```python
from build123d import *

# Parameters (mm, degrees)
SKETCH020_W             = 25.4
SKETCH020_H             = 3.175
PAD005_DEPTH            = 25.4
SKETCH001_W             = 28.575
SKETCH001_H             = 10.16
PAD006_DEPTH            = 1.81
PAD006_DEPTH_BACK       = 4.445
POCKET004_DEPTH         = 9.525
POCKET005_DEPTH         = 12.7
CHAMFER_SIZE            = 1.8034
SKETCH023_R             = 3.2512
POCKET006_DEPTH         = 4.446
PAD007_DEPTH            = 10.795
FILLET_R                = 5.08
BODY003_ROLL_ANGLE      = 90
BODY003_PLACEMENT_ANGLE = 90


with BuildPart() as part:
    # Sketch020 → Pad005 (new body)
    with BuildSketch(Plane.XY):
        with Locations((-12.7, 1.5875)):
            Rectangle(SKETCH020_W, SKETCH020_H)
    extrude(amount=PAD005_DEPTH)

    # Sketch001 (on Face1 of Pad005) → Pad006 (join, two sides)
    with BuildSketch(Plane(origin=(0, 3.175, 0), x_dir=(-1, 0, 0), z_dir=(0, 1, 0))) as pad006_sk:
        with Locations((-14.2875, 12.7)):
            Rectangle(SKETCH001_W, SKETCH001_H)
    extrude(amount=PAD006_DEPTH)
    extrude(pad006_sk.sketch, amount=-PAD006_DEPTH_BACK)

    # Sketch021 (on Face13 of Pad006) → Pocket004 (cut)
    with BuildSketch(Plane.YZ.offset(28.575)):
        Polygon((9.150137, 19.05), (2.800137, 12.7), (9.150137, 6.35), align=None)
    extrude(amount=-POCKET004_DEPTH, mode=Mode.SUBTRACT)

    # Sketch022 (on Face16 of Pocket004) → Pocket005 (cut)
    with BuildSketch(Plane.YZ.offset(19.05)):
        with BuildLine():
            ThreePointArc((4.08, 14.732), (2.048, 12.7), (4.08, 10.668))
            Line((4.985, 10.668), (4.08, 10.668))
            Line((4.985, 14.732), (4.985, 10.668))
            Line((4.08, 14.732), (4.985, 14.732))
        make_face()
    extrude(amount=-POCKET005_DEPTH, mode=Mode.SUBTRACT)

    # Chamfer
    chamfer_edges = [part.edges().sort_by_distance(p)[0] for p in [
        (0, 4.985, 12.7),
    ]]
    chamfer(chamfer_edges, length=CHAMFER_SIZE)

    # Sketch023 (on Face4 of Chamfer) → Pocket006 (cut, through all)
    with BuildSketch(Plane(origin=(0, 3.175, 0), x_dir=(-1, 0, 0), z_dir=(0, 1, 0))):
        with Locations((12.7, 12.7)):
            Circle(SKETCH023_R)
    extrude(amount=-POCKET006_DEPTH, mode=Mode.SUBTRACT)

    # Sketch024 (on Face4 of Pocket006) → Pad007 (join)
    with BuildSketch(Plane(origin=(0, 3.175, 0), x_dir=(-1, 0, 0), z_dir=(0, 1, 0))):
        Polygon((0, 0), (-3.175, 0), (-3.175, 28.575), (25.4, 28.575), (25.4, 25.4), (0, 25.4), align=None)
    extrude(amount=-PAD007_DEPTH)

    # Fillet
    fillet_edges = [part.edges().sort_by_distance(p)[0] for p in [
        (3.175, -1.27, 12.7),
    ]]
    fillet(fillet_edges, radius=FILLET_R)


with BuildPart() as part_1:
    # Body003 roll: moved
    add(part.part.rotate(Axis((0, 0, 0), (1, 0, 0)), BODY003_ROLL_ANGLE))


with BuildPart() as part_2:
    # Body003 placement: moved
    add(part_1.part.moved(Location((-58.73, -42.01, 0))).rotate(Axis((-58.73, -42.01, 0), (0, 0, 1)), BODY003_PLACEMENT_ANGLE))


solid = part_2.part
```
Input: part model. Units: mm. Frame: model coordinates. A direction names the side the tool comes from. Coordinates: 2 decimals unless noted, no trailing zeros. Order: outer loops, then holes, each group sorted by start corner. A loop starts at its lowest first (then second) coordinate and runs counter-clockwise, first axis right, second up. Notation, with made-up numbers: (34.5, 60) - (57.5, 60) arc R25 cw to (57.5, 95) - close; hole circle Ø9 at (57, 61). An arc over 180 degrees is marked (long way). Put each result on its own line as item: value.
1. Line query: line 1 along X through (y, z) = (-54.71, 1.15) (3 decimals); line 2 along Z through (x, y) = (-39.75, -54) (3 decimals); line 3 along X through (y, z) = (-49, -1) (3 decimals). Output: solid intervals per line, ascending.
Report:
line 1: x = -58.73 to -49.281, -42.779 to -30.155
line 2: z = 0 to 3.175
line 3: x = -33.33 to -30.155
2. Cut plane D-D on z = -5.75. Return the cut outline in (x, y) (3 decimals).
Report:
outline: (-58.73, -42.01) - (-33.33, -42.01) - (-33.33, -67.41) - (-30.155, -67.41) - (-30.155, -38.835) - (-40.95, -38.835) - (-40.95, -38.799) - (-51.11, -38.799) - (-51.11, -38.835) - (-58.73, -38.835) - close
3. Draft query along Y for faces 4 (the face through (-45, -38.835, -7)), 5 (the face through (-45.99, -29.22, 2.05)), 6 (the face through (-45.5, -22.96, 3.1)), 7 (the face through (-33.33, -55, -4)). Return one class per face: pulls with the +Y half, pulls with the -Y half, needs draft (parallel to the pull), parting line crosses it, or undercut.
Report:
face 4: pulls with the +Y half
face 5: undercut
face 6: undercut
face 7: needs draft
4. Cut plane C-C on x = -37.25. Return the cut outline in (y, z) (3 decimals).
Report:
outline: (-67.41, 0) - (-42.01, 0) - (-42.01, -7.62) - (-38.835, -7.62) - (-38.835, 3.175) - (-67.41, 3.175) - close
5. Cut plane A-A on y = -54.71. Return the cut outline in (x, z) (3 decimals).
Report:
outline: (-58.73, 0) - (-49.281, 0) - (-49.281, 3.175) - (-58.73, 3.175) - close; (-42.779, 0) - (-33.33, 0) - (-33.33, -7.62) - (-30.155, -7.62) - (-30.155, 3.175) - (-42.779, 3.175) - close
6. Contact query for flat-ended pins moving along their axis: pin 1 Ø2 at (y, z) = (-35.5, 1.5) entering from +X; pin 2 Ø2 at (x, z) = (-37.5, -0.5) entering from +Y (3 decimals); pin 3 Ø5 at (x, y) = (-47, -19) entering from -Z; pin 4 Ø5 at (x, y) = (-46.03, -54.71) entering from +Z. Output: stop coordinate, or through.
Report:
pin 1: stops at x = -40.95
pin 2: stops at y = -38.835
pin 3: stops at z = -1.27
pin 4: passes through
7. Cut plane B-B on y = -27. Return the cut outline in (x, z) (3 decimals), then the cut area to 3 significant figures.
Report:
outline: (-51.11, -1.27) - (-40.95, -1.27) - (-40.95, 4.985) - (-43.998, 4.985) - (-43.998, 4.08) arc R2.032 cw to (-48.062, 4.08) - (-48.062, 4.985) - (-51.11, 4.985) - close
area: 53.4 mm2
8. Reachability of faces 1 (the face through (-46, -23, -1.27)), 2 (the face through (-47.11, -18.13, 3.88)), 3 (the face through (-46, -42.01, -4)) from +Z, -Z, +X, -X, +Y, -Y: full face, straight path, thin tool, end or side. Return the list, or none.
Report:
face 1: -Z, +X, -X, +Y
face 2: +Z, +Y
face 3: -Z, -X, -Y
